Here's the drawing with two shaded views (mm, measured from the low corner). I have some questions. Give positions to 0.01 mm unless a question says otherwise; leave off trailing zeros. Write each loop counter-clockwise with the first axis right and the second up, starting at its lowest first coordinate (ties: lowest second). Pieces come first, ordered by that corner, then holes.
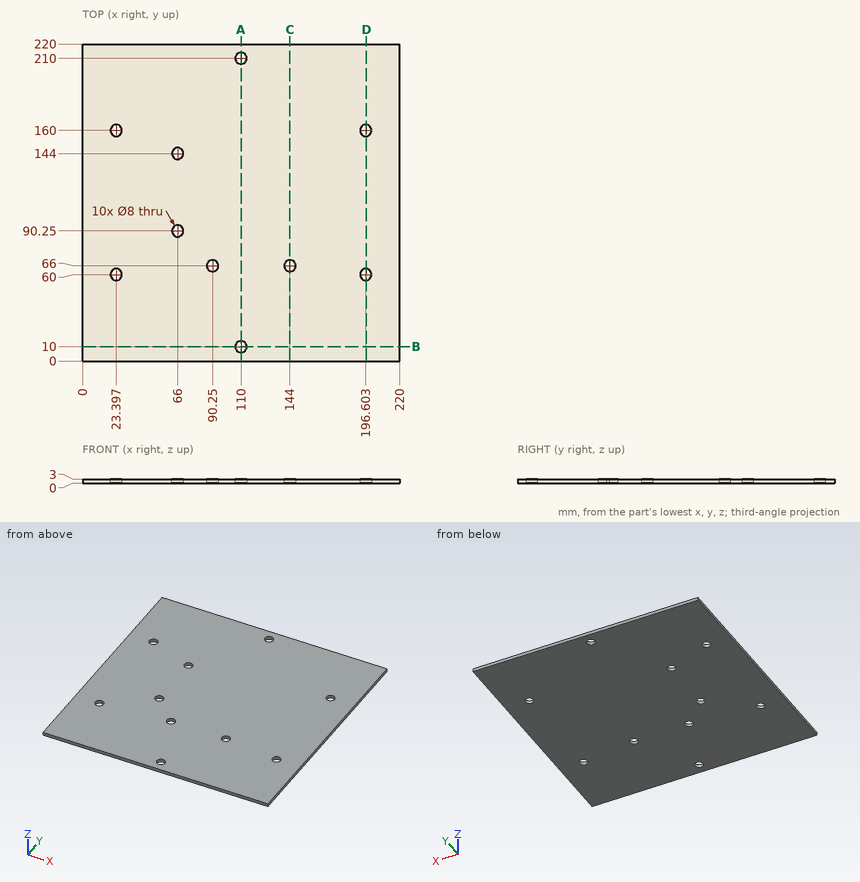
(1) Will this pin go through, and if not, where does the flat tip stop? P1, Ø6.5, axis at x = 196.6, y = 160, coming from the -Z side.
Returned:
P1: passes through
(2) Imagine slicing it at B-B, the plane y = 10. Write out the boundary of the cut face in (x, z).
Returned:
outline: (0, 0) - (106, 0) - (106, 3) - (0, 3) - close; (114, 0) - (220, 0) - (220, 3) - (114, 3) - close
(3) Imagine slicing it at D-D, the plane x = 197. Write out the boundary of the cut face in (y, z).
Returned:
outline: (0, 0) - (56.02, 0) - (56.02, 3) - (0, 3) - close; (63.98, 0) - (156.02, 0) - (156.02, 3) - (63.98, 3) - close; (163.98, 0) - (220, 0) - (220, 3) - (163.98, 3) - close
(4) Imagine slicing it at A-A, the plane x = 110. Write out the boundary of the cut face in (y, z), plus the area to 3 significant figures.
Returned:
outline: (0, 0) - (6, 0) - (6, 3) - (0, 3) - close; (14, 0) - (206, 0) - (206, 3) - (14, 3) - close; (214, 0) - (220, 0) - (220, 3) - (214, 3) - close
area: 612 mm2
(5) Imagine slicing it at C-C, the plane x = 144. Write out the boundary of the cut face in (y, z), plus the area to 3 significant figures.
Returned:
outline: (0, 0) - (62, 0) - (62, 3) - (0, 3) - close; (70, 0) - (220, 0) - (220, 3) - (70, 3) - close
area: 636 mm2
(6) If I drill on L1, parallel to Y at x = 66, z = 2.35; L2, parallel to X at y = 210, z = 0.8; L3, parallel to X at y = 144, z = 1.85, over which ranges is the centre line in solid material (lowest first)?
Returned:
L1: y = 0 to 86.25, 94.25 to 140, 148 to 220
L2: x = 0 to 106, 114 to 220
L3: x = 0 to 62, 70 to 220
